Build history of the part. All positions in model axes, mm. Face numbers are marked on the shaded views. A direction names the side the tool comes from. Round coordinates to 2 decimals unless told otherwise and drop trailing zeros. Write each loop counter-clockwise with the first axis right and the second up, starting at its lowest first coordinate (ties: lowest second). Pieces come first, ordered by that corner, then holes. Notation, with made-up numbers: (10.5, 16) -> (28.5, 16) arc R13 cw to (28.5, 22) -> close; hole circle Ø1 at (-15.5, 50.5). An arc over 180 degrees is marked (long way). Return JSON: item names as keys, results as strings.
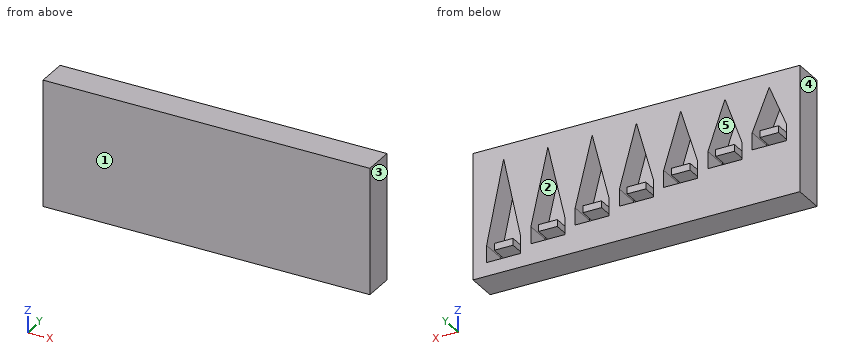
from build123d import *

# Parameters (mm, degrees)
FLAPS_W               = 96
FLAPS_H               = 37
BOSS_EXTRUDE1_DEPTH   = 7.5
FLAPS_W_2             = 5.5
FLAPS_H_2             = 2
BOSS_EXTRUDE1_2_DEPTH = 7.5
BOSS_EXTRUDE1_3_DEPTH = 7.5
BOSS_EXTRUDE1_4_DEPTH = 7.5
BOSS_EXTRUDE1_5_DEPTH = 7.5
BOSS_EXTRUDE1_6_DEPTH = 7.5
BOSS_EXTRUDE1_7_DEPTH = 7.5
BOSS_EXTRUDE1_8_DEPTH = 7.5
SKETCH2_W             = 96
SKETCH2_H             = 37
BOSS_EXTRUDE2_DEPTH   = 1.5


with BuildPart() as part:
    # Flaps → Boss-Extrude1 (new body)
    with BuildSketch(Plane(origin=(0, 0, 0), x_dir=(1, 0, 0), z_dir=(0, 1, 0))):
        with Locations((39, 14.5)):
            Rectangle(FLAPS_W, FLAPS_H)
        Polygon((78, 0), (83, 24), (83, 29), (73, 29), (73, 24), align=None, mode=Mode.SUBTRACT)
        Polygon((65, 0), (70, 22), (70, 27), (60, 27), (60, 22), align=None, mode=Mode.SUBTRACT)
        Polygon((52, 0), (57, 20), (57, 25), (47, 25), (47, 20), align=None, mode=Mode.SUBTRACT)
        Polygon((39, 0), (44, 18), (44, 23), (34, 23), (34, 18), align=None, mode=Mode.SUBTRACT)
        Polygon((26, 0), (31, 16), (31, 21), (21, 21), (21, 16), align=None, mode=Mode.SUBTRACT)
        Polygon((13, 0), (18, 14), (18, 19), (8, 19), (8, 14), align=None, mode=Mode.SUBTRACT)
        Polygon((0, 0), (5, 12), (5, 17), (-5, 17), (-5, 12), align=None, mode=Mode.SUBTRACT)
    extrude(amount=BOSS_EXTRUDE1_DEPTH)



with BuildPart() as body_2:
    # Flaps → Boss-Extrude1 2 (new body)
    with BuildSketch(Plane(origin=(0, 0, 0), x_dir=(1, 0, 0), z_dir=(0, 1, 0))):
        with Locations((0, 13)):
            Rectangle(FLAPS_W_2, FLAPS_H_2)
    extrude(amount=BOSS_EXTRUDE1_2_DEPTH)


with BuildPart() as body_3:
    # Flaps → Boss-Extrude1 3 (new body)
    with BuildSketch(Plane(origin=(0, 0, 0), x_dir=(1, 0, 0), z_dir=(0, 1, 0))):
        with Locations((13, 15)):
            Rectangle(FLAPS_W_2, FLAPS_H_2)
    extrude(amount=BOSS_EXTRUDE1_3_DEPTH)


with BuildPart() as body_4:
    # Flaps → Boss-Extrude1 4 (new body)
    with BuildSketch(Plane(origin=(0, 0, 0), x_dir=(1, 0, 0), z_dir=(0, 1, 0))):
        with Locations((26, 17)):
            Rectangle(FLAPS_W_2, FLAPS_H_2)
    extrude(amount=BOSS_EXTRUDE1_4_DEPTH)


with BuildPart() as body_5:
    # Flaps → Boss-Extrude1 5 (new body)
    with BuildSketch(Plane(origin=(0, 0, 0), x_dir=(1, 0, 0), z_dir=(0, 1, 0))):
        with Locations((39, 19)):
            Rectangle(FLAPS_W_2, FLAPS_H_2)
    extrude(amount=BOSS_EXTRUDE1_5_DEPTH)


with BuildPart() as body_6:
    # Flaps → Boss-Extrude1 6 (new body)
    with BuildSketch(Plane(origin=(0, 0, 0), x_dir=(1, 0, 0), z_dir=(0, 1, 0))):
        with Locations((52, 21)):
            Rectangle(FLAPS_W_2, FLAPS_H_2)
    extrude(amount=BOSS_EXTRUDE1_6_DEPTH)


with BuildPart() as body_7:
    # Flaps → Boss-Extrude1 7 (new body)
    with BuildSketch(Plane(origin=(0, 0, 0), x_dir=(1, 0, 0), z_dir=(0, 1, 0))):
        with Locations((65, 23)):
            Rectangle(FLAPS_W_2, FLAPS_H_2)
    extrude(amount=BOSS_EXTRUDE1_7_DEPTH)


with BuildPart() as body_8:
    # Flaps → Boss-Extrude1 8 (new body)
    with BuildSketch(Plane(origin=(0, 0, 0), x_dir=(1, 0, 0), z_dir=(0, 1, 0))):
        with Locations((78, 25)):
            Rectangle(FLAPS_W_2, FLAPS_H_2)
    extrude(amount=BOSS_EXTRUDE1_8_DEPTH)


with BuildPart() as part_1:
    add(part.part)

    add(body_2.part)  # Boss-Extrude2 merges body 2

    add(body_3.part)  # Boss-Extrude2 merges body 3

    add(body_4.part)  # Boss-Extrude2 merges body 4

    add(body_5.part)  # Boss-Extrude2 merges body 5

    add(body_6.part)  # Boss-Extrude2 merges body 6

    add(body_7.part)  # Boss-Extrude2 merges body 7

    add(body_8.part)  # Boss-Extrude2 merges body 8
    # Sketch2 → Boss-Extrude2 (add)
    with BuildSketch(Plane.XZ):
        with Locations((39, -14.5)):
            Rectangle(SKETCH2_W, SKETCH2_H)
    extrude(amount=BOSS_EXTRUDE2_DEPTH)


solid = part_1.part
Q1. Saw through at A-A on y = 1. Count the separate pieces of the cut face and the enclosed holes in it, then the cut area to 3 significant figures.
Verdict:
{"separate pieces": "8", "enclosed holes": "7", "area": "2,650 mm²"}
Q2. 3-axis set-ups, long thin cutter, end or side, ignore diameter. For the marked faces 4 and 5: which of +Z, -Z, +X, -X, +Y, -Y reach the whole face in a straight line?
Verdict:
{"face 4": "+Z, -Z, -X, +Y, -Y", "face 5": "+Y"}
Q3. Two-plate mould, pull along X, no slides. Class the marked faces 1, 2 and 3: +X half, -X half, draft (parallel to the pull), parting line (faces both ways), or undercut.
Verdict:
{"face 1": "draft", "face 2": "undercut", "face 3": "+X half"}
Q4. Wall check: L1, parallel to X at y = 0.5, z = -25.5; L2, parallel to Y at x = 63, z = -13.5; L3, parallel to Z at x = 1, y = 2.5. Give the ranges that are in metal, low to high.
Verdict:
{"L1": "x = -9 to 60, 70 to 73, 75.25 to 80.75, 83 to 87", "L2": "y = -1.5 to 0", "L3": "z = -33 to -17, -14 to -12, -2.4 to 4"}
Q5. Saw through at B-B on x = 53. List the corners of the cut face in (y, z).
Verdict:
{"outline": "(-1.5, -33) -> (7.5, -33) -> (7.5, -25) -> (0, -25) -> (0, -22) -> (7.5, -22) -> (7.5, -20) -> (0, -20) -> (0, -4) -> (7.5, -4) -> (7.5, 4) -> (-1.5, 4) -> close"}
Q6. Pin check, flat tips, straight feed: pin 1 Ø4 at (x, z) = (24.5, -12.5) entering from +Y; pin 2 Ø5 at (x, z) = (41.5, -17) entering from +Y. Stop position of each tip, or through.
Verdict:
{"pin 1": "stops at y = 0", "pin 2": "stops at y = 7.5"}
